from build123d import *

# Parameters (mm, degrees)
BASE_FLANGE1_DEPTH      = 13.5
SKETCH5_R               = 4
SKETCH5_R_2             = 1.05
CUT_EXTRUDE1_DEPTH      = 10
CUT_EXTRUDE2_DEPTH      = 102.5603269
CUT_EXTRUDE2_DEPTH_BACK = 102.5603269
CUT_EXTRUDE3_DEPTH      = 104.495168969
CUT_EXTRUDE3_DEPTH_BACK = 104.495168969
SKETCH7_R               = 1.35
FILLET1_R               = 4


# Sheet-metal steps are written as plain solids
with BuildPart() as part:
    # Sketch1 → Base-Flange1 (new, symmetric)
    with BuildSketch(Plane.XY):
        with BuildLine():
            Line((-10, 100), (-10, 2.5))
            ThreePointArc((-10, 2.5), (-9.267766953, 0.732233047), (-7.5, 0))
            Line((-7.5, 0), (7.5, 0))
            ThreePointArc((7.5, 0), (9.267766953, 0.732233047), (10, 2.5))
            Line((10, 2.5), (10, 100))
            Line((10, 100), (11.5, 100))
            Line((11.5, 100), (11.5, 2.5))
            ThreePointArc((11.5, 2.5), (10.328427125, -0.328427125), (7.5, -1.5))
            Line((7.5, -1.5), (-7.5, -1.5))
            ThreePointArc((-7.5, -1.5), (-10.328427125, -0.328427125), (-11.5, 2.5))
            Line((-11.5, 2.5), (-11.5, 100))
            Line((-11.5, 100), (-10, 100))
        make_face()
    extrude(amount=BASE_FLANGE1_DEPTH, both=True)

    # Sketch5 → Cut-Extrude1 (cut)
    with BuildSketch(Plane(origin=(0, 0, 0), x_dir=(1, 0, 0), z_dir=(0, 1, 0))):
        with Locations(Location((0, 0, 0), (0, 0, 270))):
            Circle(SKETCH5_R)
        with Locations(Location((-5.656854249, 5.656854249, 0), (0, 0, 270))):
            Circle(SKETCH5_R_2)
        with Locations(Location((0, 8, 0), (0, 0, 270))):
            Circle(SKETCH5_R_2)
        with Locations(Location((5.656854249, 5.656854249, 0), (0, 0, 270))):
            Circle(SKETCH5_R_2)
        with Locations(Location((5.656854249, -5.656854249, 0), (0, 0, 270))):
            Circle(SKETCH5_R_2)
        with Locations(Location((0, -8, 0), (0, 0, 270))):
            Circle(SKETCH5_R_2)
        with Locations(Location((-5.656854249, -5.656854249, 0), (0, 0, 270))):
            Circle(SKETCH5_R_2)
    extrude(amount=-CUT_EXTRUDE1_DEPTH, mode=Mode.SUBTRACT)

    # Sketch6 → Cut-Extrude2 (cut, two sides: drawn at the far end of the back side and taken through both)
    with BuildSketch(Plane(origin=(0, 0, 0), x_dir=(0, 0, -1), z_dir=(1, 0, 0)).offset(-CUT_EXTRUDE2_DEPTH_BACK)):
        Polygon((-1.5, 100), (-1.5, 27), (-13.5, 15), (-13.5, 100), align=None)
    extrude(amount=CUT_EXTRUDE2_DEPTH + CUT_EXTRUDE2_DEPTH_BACK, mode=Mode.SUBTRACT)

    # Sketch7 → Cut-Extrude3 (cut, two sides: drawn at the far end of the back side and taken through both)
    with BuildSketch(Plane(origin=(11.5, 0, 0), x_dir=(0, 0, -1), z_dir=(1, 0, 0)).offset(-CUT_EXTRUDE3_DEPTH_BACK)):
        with Locations(Location((6, 95, 0), (0, 0, 90))):
            Circle(SKETCH7_R)
        with Locations(Location((6, 85, 0), (0, 0, 90))):
            Circle(SKETCH7_R)
        with Locations(Location((6, 75, 0), (0, 0, 90))):
            Circle(SKETCH7_R)
        with Locations(Location((6, 65, 0), (0, 0, 90))):
            Circle(SKETCH7_R)
    extrude(amount=CUT_EXTRUDE3_DEPTH + CUT_EXTRUDE3_DEPTH_BACK, mode=Mode.SUBTRACT)

    # Fillet1
    fillet1_edges = [part.edges().sort_by_distance(p)[0] for p in [
        (-10.75, 27, 1.5),
        (-10.75, 100, 1.5),
        (-10.75, 15, 13.5),
        (-10.75, 100, -13.5),
        (10.75, 27, 1.5),
        (10.75, 15, 13.5),
        (10.75, 100, 1.5),
        (10.75, 100, -13.5),
    ]]
    fillet(fillet1_edges, radius=FILLET1_R)


solid = part.part
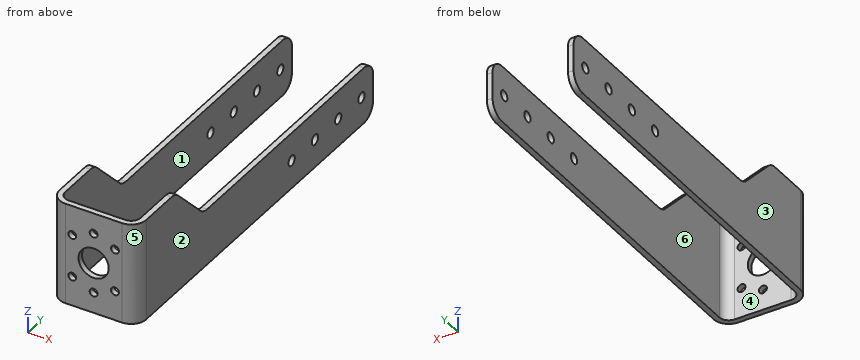
Geometry: final body of the model. Coordinates: model frame, mm. Face numbers are marked on the shaded views. A direction names the side the tool comes from. Coordinates: 2 decimals unless noted, no trailing zeros. Order: outer loops, then holes, each group sorted by start corner. A loop starts at its lowest first (then second) coordinate and runs counter-clockwise, first axis right, second up.
(1) First-contact query: pin 1 (1.6 mm diameter, centred on x = 10.5, y = 62.5, fed in from +Z); pin 2 (1.7 mm diameter, centred on x = 0, z = 8, fed in from +Y); pin 3 (4 mm diameter, centred on x = -3.5, z = 7, fed in from +Y); pin 4 (3 mm diameter, centred on y = 65, z = -6, fed in from -X). Flat tips, straight axial feed; report the tip coordinate or a pass-through.
(2) Section query B-B (z = 8). Return the cut outline in (x, y).
(3) Access query for the marked faces 5 and 6. Directions: +Z, -Z, +X, -X, +Y, -Y. A direction counts if a zero-diameter tool reaches every point of the face in a straight line with its end or side. Return the directions, or none.
(4) Material intervals for probe 1 along X at (y, z) = (29, -6); probe 2 along Z at (x, y) = (10.9, 95); probe 3 along Y at (x, z) = (7.25, 8.5), sorted ascending.
(5) Section query A-A (y = 20.5). Return the cut outline in (x, z), plus the area to 3 significant figures.
(6) Draft query along X for the marked faces 1, 2, 3 and 4. Return one class per face: pulls with the +X half, pulls with the -X half, needs draft (parallel to the pull), parting line crosses it, or undercut.
(7) Section query C-C (y = 85). Return the cut outline in (x, z), plus the area to 3 significant figures.
(8) Section query D-D (x = 0). Return the cut outline in (y, z).
Solution:
1. pin 1: stops at z = 1.5
1. pin 2: passes through
1. pin 3: stops at y = 0
1. pin 4: stops at x = -11.5
2. outline: (-11.5, 2.5) arc R4 ccw to (-7.5, -1.5) - (-1.05, -1.5) - (-1.05, 0) - (-7.5, 0) arc R2.5 cw to (-10, 2.5) - (-10, 20.5) - (-11.5, 20.5) - close; (1.05, -1.5) - (7.5, -1.5) arc R4 ccw to (11.5, 2.5) - (11.5, 20.5) - (10, 20.5) - (10, 2.5) arc R2.5 cw to (7.5, 0) - (1.05, 0) - close
3. face 5: +Z, -Z, +X, -Y
3. face 6: +Z, -Z, +Y
4. probe 1: x = -11.5 to -10, 10 to 11.5
4. probe 2: z = -13.5 to -7.35, -4.65 to 1.5
4. probe 3: y = -1.5 to 0
5. outline: (-11.5, -13.5) - (-10, -13.5) - (-10, 8) - (-11.5, 8) - close; (10, -13.5) - (11.5, -13.5) - (11.5, 8) - (10, 8) - close
5. area: 64.5 mm2
6. face 1: undercut
6. face 2: pulls with the +X half
6. face 3: pulls with the -X half
6. face 4: undercut
7. outline: (-11.5, -13.5) - (-10, -13.5) - (-10, -7.35) - (-11.5, -7.35) - close; (-11.5, -4.65) - (-10, -4.65) - (-10, 1.5) - (-11.5, 1.5) - close; (10, -13.5) - (11.5, -13.5) - (11.5, -7.35) - (10, -7.35) - close; (10, -4.65) - (11.5, -4.65) - (11.5, 1.5) - (10, 1.5) - close
7. area: 36.9 mm2
8. outline: (-1.5, -13.5) - (0, -13.5) - (0, -9.05) - (-1.5, -9.05) - close; (-1.5, -6.95) - (0, -6.95) - (0, -4) - (-1.5, -4) - close; (-1.5, 4) - (0, 4) - (0, 6.95) - (-1.5, 6.95) - close; (-1.5, 9.05) - (0, 9.05) - (0, 13.5) - (-1.5, 13.5) - close
